from build123d import *

# Parameters (mm, degrees)
F0_R     = 9.65
F0_R_2   = 7.575
F1_DEPTH = 20
F2_R     = 7.575
F3_DEPTH = 15
F4_R     = 1.1
F5_DEPTH = 5.001


with BuildPart() as f1:
    # F0 (on Top) → F1 (new body)
    with BuildSketch(Plane.XY):
        Circle(F0_R)
        Circle(F0_R_2, mode=Mode.SUBTRACT)
        Circle(F0_R_2)
    extrude(amount=F1_DEPTH)

    # F2 (on face) → F3 (cut)
    with BuildSketch(Plane(origin=(0, 0, 0), x_dir=(1, 0, 0), z_dir=(0, 0, -1))):
        Circle(F2_R)
    extrude(amount=-F3_DEPTH, mode=Mode.SUBTRACT)

    # F4 (on face) → F5 (cut, through all)
    with BuildSketch(Plane(origin=(0, 0, 15), x_dir=(1, 0, 0), z_dir=(0, 0, -1))):
        with Locations((-0.039568, 1.999609)):
            Circle(F4_R)
        with Locations((0.039568, -1.999609)):
            Circle(F4_R)
    extrude(amount=-F5_DEPTH, mode=Mode.SUBTRACT)


solid = f1.part
Can you work these out from the model? Positions are in its coordinate system, mm. A direction names the side the tool comes from. Give positions to 0.01 mm unless a question says otherwise; leave off trailing zeros. Loops run counter-clockwise (first coordinate to the right, second up) from the corner with the lowest first, then second, coordinate; pieces in that order, holes last. Notation, with made-up numbers: (84, -2) -> (100, -2) arc R23 ccw to (100, 18) -> close; hole circle Ø4 at (33, -26). An arc over 180 degrees is marked (long way). Use one line per item in the form item = value.
1) Will these pins go through, and if not, where does the flat tip stop? pin 1 (2 mm diameter, centred on y = 3, z = 8, fed in from +X); pin 2 (1.3 mm diameter, centred on x = -0.04, y = -2, fed in from -Z); pin 3 (6 mm diameter, centred on y = -6, z = 4.5, fed in from -X); pin 4 (2 mm diameter, centred on x = 0, y = -4.5, fed in from -Z).
Answers:
pin_1 = 9.44
pin_2 = through
pin_3 = -9.17
pin_4 = 15
2) If we section it at B-B (x = 0): Please give me the cut outline in (y, z) (3 decimals).
Answers:
outline = (-9.65, 0) -> (-7.575, 0) -> (-7.575, 15) -> (-3.099, 15) -> (-3.099, 20) -> (-9.65, 20) -> close; (-0.9, 15) -> (0.9, 15) -> (0.9, 20) -> (-0.9, 20) -> close; (3.099, 15) -> (7.575, 15) -> (7.575, 0) -> (9.65, 0) -> (9.65, 20) -> (3.099, 20) -> close
3) I need wall thicknesses on line 1 along Y through (x, z) = (0, 11) (3 decimals); line 2 along Z through (x, y) = (-2.5, -4); line 3 along X through (y, z) = (-5.5, 13). Which ranges of each line are inside material? Lowest first, please.
Answers:
line_1 = -9.65 to -7.575, 7.575 to 9.65
line_2 = 15 to 20
line_3 = -7.93 to -5.21, 5.21 to 7.93
4) If we section it at D-D (x = 7): Please give me the cut outline in (y, z), plus the area to 3 significant figures.
Answers:
outline = (-6.64, 0) -> (-2.89, 0) -> (-2.89, 15) -> (2.89, 15) -> (2.89, 0) -> (6.64, 0) -> (6.64, 20) -> (-6.64, 20) -> close
area = 179 mm²
5) If we section it at A-A (y = 0): Please give me the cut outline in (x, z) (3 decimals).
Answers:
outline = (-9.65, 0) -> (-7.575, 0) -> (-7.575, 15) -> (7.575, 15) -> (7.575, 0) -> (9.65, 0) -> (9.65, 20) -> (-9.65, 20) -> close
6) We'd pull the mould along Y, two halves only. Please class faces 3 (the face through (9.204, 2.899, 9.86)), 4 (the face through (-6.01, 4.61, 7.4)), 5 (the face through (0, 0, 20)): released by +Y, released by -Y, zero draft, split by the parting line, or undercut.
Answers:
face_3 = split by the parting line
face_4 = undercut
face_5 = zero draft
7) If we section it at C-C (z = 2.75): Please give me the cut outline in (x, y) (3 decimals).
Answers:
outline = circle Ø19.3 at (0, 0); hole circle Ø15.15 at (0, 0)
8) For faces 1 (the face through (-6, -5, 0)), 2 (the face through (0, 0, 15)), which set-ups out of +Z, -Z, +X, -X, +Y, -Y let a thin tool reach every point of the face, with its end or its side?
Answers:
face_1 = -Z, +X, -X, +Y, -Y
face_2 = -Z
